Input: part model. Units: mm. Frame: model coordinates. A direction names the side the tool comes from. Coordinates: 2 decimals unless noted, no trailing zeros. Loops run counter-clockwise (first coordinate to the right, second up) from the corner with the lowest first, then second, coordinate; pieces in that order, holes last. Notation, with made-up numbers: M 23,-32 L 81,-32 A20 cw 81,-18 Z; hole C 34,81.5 d1. An arc over 180 degrees is marked long. Use a Markdown table: item, result. Add a question column.
1. Section A-A on z = 17.5. Output: boundary loops of the cut face in (x, y).
2. Section C-C on x = -3. Output: boundary loops of the cut face in (y, z), then the cut area to 3 significant figures.
3. Set-up query: faces 1 (the flat face through (-100, -1, 17)), 2 (the flat face through (-92.5, 0, 14)), 3 (the cylindrical face through (75.21, -36.3, 15.01)). Return all of +Z, -Z, +X, -X, +Y, -Y with unobstructed straight access to the full face (end or side cutting, diameter ignored); none if empty.
4. Section B-B on y = 36.25. Output: boundary loops of the cut face in (x, z).
5. Line query: L1, parallel to Y at x = -96.25, z = 1; L2, parallel to X at y = -36, z = 1; L3, parallel to X at y = 37, z = 17. Output: solid intervals per line, ascending. Write a range as [from, to].
6. Pin query (flat end, axial travel): pin 1 (1.5 mm diameter, centred on x = 96, y = -36, fed in from -Z). Return the tip coordinate at first contact, or that it passes through.
7. Section D-D on x = 80. Output: boundary loops of the cut face in (y, z), then the cut area to 4 significant figures.
8. Draft query along Z for faces 4 (the flat face through (-1, 1, 35)), 5 (the flat face through (-1, 40, 17)), 6 (the cylindrical face through (-52.068, 36.302, 16.459)), 7 (the cylindrical face through (-72.068, 36.302, 16.459)). Return one class per face: +Z half, -Z half, draft (parallel to the pull), parting line (faces both ways), or undercut.
```python
from build123d import *

# Parameters (mm, degrees)
CROQUIS1_W              = 200
CROQUIS1_H              = 80
SALIENTE_EXTRUIR1_DEPTH = 35
CROQUIS2_W              = 185
CROQUIS2_H              = 65
CORTAR_EXTRUIR1_DEPTH   = 27.5
CROQUIS3_R              = 8
CORTAR_EXTRUIR2_DEPTH   = 7.5
CROQUIS4_R              = 5.4
CORTAR_EXTRUIR3_DEPTH   = 7.5
CROQUIS5_R              = 2.50919292
CORTAR_EXTRUIR4_DEPTH   = 2


with BuildPart() as part:
    # Croquis1 → Saliente-Extruir1 (new body)
    with BuildSketch(Plane.XY):
        Rectangle(CROQUIS1_W, CROQUIS1_H)
    extrude(amount=SALIENTE_EXTRUIR1_DEPTH)

    # Croquis2 → Cortar-Extruir1 (cut)
    with BuildSketch(Plane(origin=(0, 0, 0), x_dir=(-1, 0, 0), z_dir=(0, 0, -1))):
        Rectangle(CROQUIS2_W, CROQUIS2_H)
    extrude(amount=-CORTAR_EXTRUIR1_DEPTH, mode=Mode.SUBTRACT)

    # Croquis3 → Cortar-Extruir2 (cut)
    with BuildSketch(Plane(origin=(0, 40, 0), x_dir=(1, 0, 0), z_dir=(0, 1, 0))):
        with Locations(Location((-80, -17.5, 0), (0, 0, 270))):
            Circle(CROQUIS3_R)
        with Locations(Location((-60, -17.5, 0), (0, 0, 270))):
            Circle(CROQUIS3_R)
        with Locations(Location((-40, -17.5, 0), (0, 0, 270))):
            Circle(CROQUIS3_R)
    extrude(amount=-CORTAR_EXTRUIR2_DEPTH, mode=Mode.SUBTRACT)

    # Croquis4 → Cortar-Extruir3 (cut)
    with BuildSketch(Plane.XZ.offset(40)):
        with Locations(Location((80, 17.5, 0), (0, 0, 270))):
            Circle(CROQUIS4_R)
    extrude(amount=-CORTAR_EXTRUIR3_DEPTH, mode=Mode.SUBTRACT)

    # Croquis5 → Cortar-Extruir4 (cut)
    with BuildSketch(Plane(origin=(0, 0, 0), x_dir=(-1, 0, 0), z_dir=(0, 0, -1))):
        with Locations((96.25, -36.25)):
            Circle(CROQUIS5_R)
        with Locations((96.25, 36.25)):
            Circle(CROQUIS5_R)
        with Locations((-96.25, 36.25)):
            Circle(CROQUIS5_R)
        with Locations((-96.25, -36.25)):
            Circle(CROQUIS5_R)
    extrude(amount=-CORTAR_EXTRUIR4_DEPTH, mode=Mode.SUBTRACT)


solid = part.part
```
Answers below:
| question | item | result |
|---|---|---|
| 1 | outline | M -100,-40 L 74.6,-40 L 74.6,-32.5 L -92.5,-32.5 L -92.5,32.5 L -88,32.5 L -88,40 L -100,40 Z; M -72,32.5 L -68,32.5 L -68,40 L -72,40 Z; M -52,32.5 L -48,32.5 L -48,40 L -52,40 Z; M -32,32.5 L 92.5,32.5 L 92.5,-32.5 L 85.4,-32.5 L 85.4,-40 L 100,-40 L 100,40 L -32,40 Z |
| 2 | outline | M -40,0 L -32.5,0 L -32.5,27.5 L 32.5,27.5 L 32.5,0 L 40,0 L 40,35 L -40,35 Z |
| 2 | area | 1,010 mm² |
| 3 | face 1 | +Z, -Z, -X, +Y, -Y |
| 3 | face 2 | -Z |
| 3 | face 3 | -Y |
| 4 | outline | M -100,0 L -98.76,0 L -98.76,2 L -93.74,2 L -93.74,0 L 93.74,0 L 93.74,2 L 98.76,2 L 98.76,0 L 100,0 L 100,35 L -100,35 Z; hole C -80,17.5 d16; hole C -60,17.5 d16; hole C -40,17.5 d16 |
| 5 | L1 | y = [-40, -38.76], [-33.74, 33.74], [38.76, 40] |
| 5 | L2 | x = [-100, -98.75], [-93.75, 93.75], [98.75, 100] |
| 5 | L3 | x = [-100, -87.98], [-72.02, -67.98], [-52.02, -47.98], [-32.02, 100] |
| 6 | pin 1 | stops at z = 2 |
| 7 | outline | M -40,0 L -32.5,0 L -32.5,12.1 L -40,12.1 Z; M -40,22.9 L -32.5,22.9 L -32.5,27.5 L 32.5,27.5 L 32.5,0 L 40,0 L 40,35 L -40,35 Z |
| 7 | area | 931.5 mm² |
| 8 | face 4 | +Z half |
| 8 | face 5 | draft |
| 8 | face 6 | undercut |
| 8 | face 7 | undercut |
